Can you work these out from the drawing? Everything is in mm from the part's minimum corner. Coordinates: 2 decimals unless noted, no trailing zeros. Write each loop counter-clockwise with the first axis right and the second up, starting at its lowest first coordinate (ties: lowest second). Pieces come first, ordered by that corner, then holes.
(1) Imagine slicing it at B-B, the plane y = 1.5. List the corners of the cut face in (x, z) for me.
(2) Imagine slicing it at C-C, the plane x = 102. List the corners of the cut face in (y, z) for me.
(3) Imagine slicing it at A-A, the plane x = 56. List the corners of the cut face in (y, z) for me.
(4) Please list where these lines run through material, in increasing order: probe 1 along Z at (x, y) = (56, 1.75); probe 2 along Z at (x, y) = (7, 1.9); probe 3 along X at (y, z) = (0.85, 60).
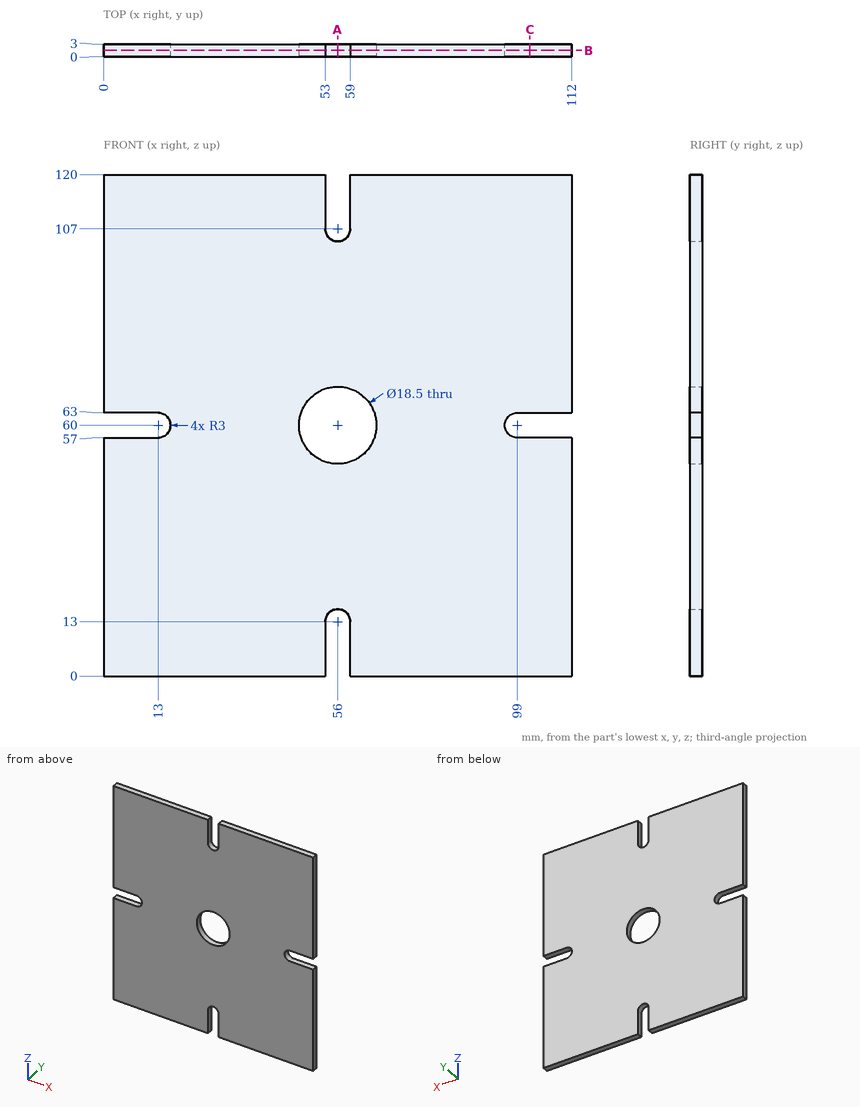
Recorded:
1. outline: (0, 0) - (53, 0) - (53, 13) arc R3 cw to (59, 13) - (59, 0) - (112, 0) - (112, 57) - (99, 57) arc R3 cw to (99, 63) - (112, 63) - (112, 120) - (59, 120) - (59, 107) arc R3 cw to (53, 107) - (53, 120) - (0, 120) - (0, 63) - (13, 63) arc R3 cw to (13, 57) - (0, 57) - close; hole circle Ø18.5 at (56, 60)
2. outline: (0, 0) - (3, 0) - (3, 57) - (0, 57) - close; (0, 63) - (3, 63) - (3, 120) - (0, 120) - close
3. outline: (0, 16) - (3, 16) - (3, 50.75) - (0, 50.75) - close; (0, 69.25) - (3, 69.25) - (3, 104) - (0, 104) - close
4. probe 1: z = 16 to 50.75, 69.25 to 104
4. probe 2: z = 0 to 57, 63 to 120
4. probe 3: x = 16 to 46.75, 65.25 to 96
